Could you check a few things on this drawing? It's one solid part, dimensions in mm from its lowest x, y, z. A direction names the side the tool comes from. Coordinates: 2 decimals unless noted, no trailing zeros. Write each loop counter-clockwise with the first axis right and the second up, starting at its lowest first coordinate (ties: lowest second). Pieces come first, ordered by that corner, then holes.
Item 1: I'm going to push flat-ended pins straight in: P1, Ø2, axis at x = 21, z = 73, coming from the -Y side; P2, Ø12, axis at x = 72.5, z = 57.5, coming from the +Y side (3 decimals); P3, Ø8, axis at y = 17, z = 28, coming from the +X side. Where does each tip first touch, or does it pass through?
Item 2: I want a section at A-A (x = 12.7). Count the separate pieces of the cut face and the enclosed holes in it, and give its area (3 significant figures).
Item 3: If we mould it in two halves opening along X, with no side actions, what happens to the marked faces 1, 2, 3 and 4? For each: pulls with the +X half, pulls with the -X half, needs draft (parallel to the pull), parting line crosses it, or undercut.
Item 4: I want a section at C-C (z = 39). Please give me the cut outline in (x, y) (3 decimals), and give its area (3 significant figures).
Item 5: For the marked faces 5 and 6, which set-ups out of +Z, -Z, +X, -X, +Y, -Y let a thin tool reach every point of the face, with its end or its side?
Item 6: Please list where these lines run through material, in increasing order: line 1 (Z direction, x = 82.55, y = 3); line 2 (Z direction, x = 17, y = 6); line 3 (Y direction, x = 74, z = 12) (3 decimals).
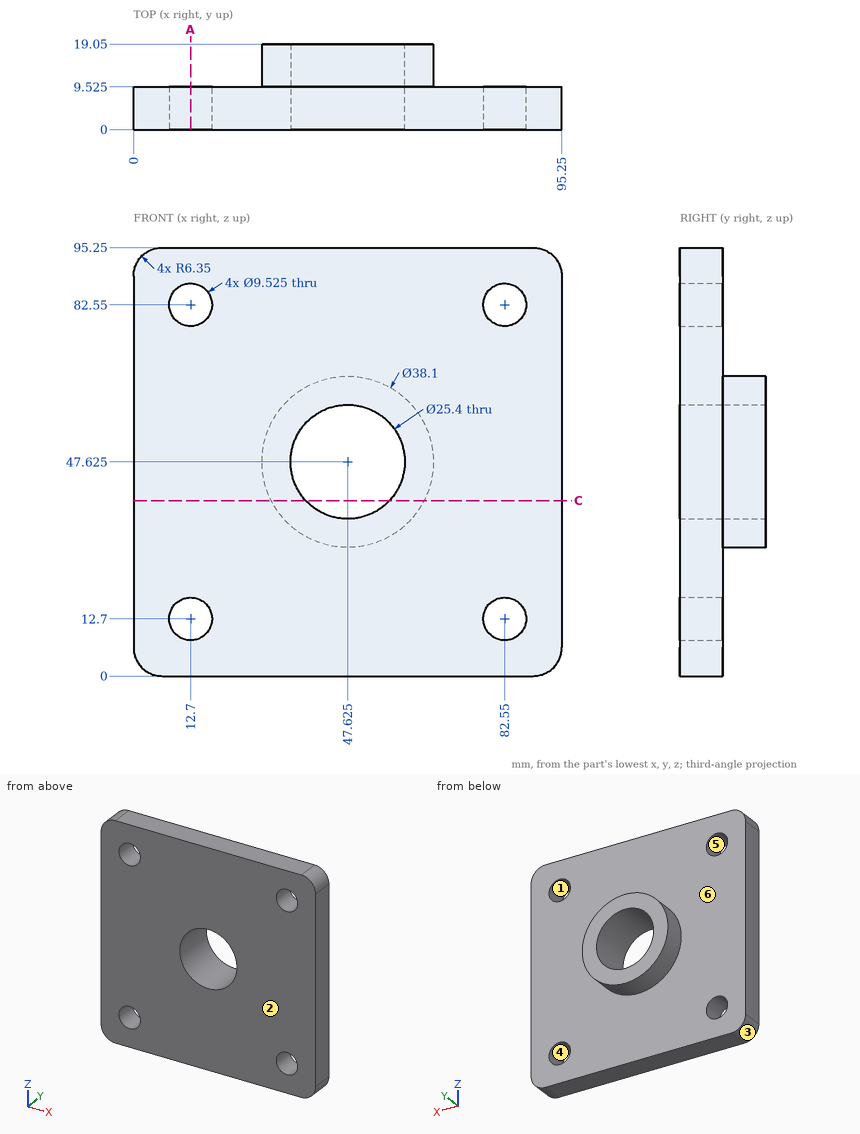
Answer:
1. P1: stops at y = 0
1. P2: stops at y = 9.525
1. P3: stops at x = 58.52
2. separate pieces: 3
2. enclosed holes: 0
2. area: 726 mm2
3. face 1: undercut
3. face 2: needs draft
3. face 3: pulls with the -X half
3. face 4: undercut
4. outline: (0, 0) - (38.303, 0) - (38.303, 19.05) - (30.639, 19.05) - (30.639, 9.525) - (0, 9.525) - close; (56.947, 0) - (95.25, 0) - (95.25, 9.525) - (64.611, 9.525) - (64.611, 19.05) - (56.947, 19.05) - close
4. area: 876 mm2
5. face 5: +Y, -Y
5. face 6: +Y
6. line 1: z = 0 to 7.94, 17.46 to 77.79, 87.31 to 95.25
6. line 2: z = 0 to 10.65, 14.75 to 80.5, 84.6 to 95.25
6. line 3: y = 0 to 9.525
